```python
from build123d import *

# Parameters (mm, degrees)
SKETCH1_R                = 16.5
BOSS_EXTRUDE1_DEPTH      = 47.5
SKETCH2_R                = 14
BOSS_EXTRUDE2_DEPTH      = 4
SKETCH4_R                = 1.6
BOSS_EXTRUDE3_DEPTH      = 8
BOSS_EXTRUDE3_DEPTH_BACK = 1
SKETCH5_R                = 1.6
BOSS_EXTRUDE4_DEPTH      = 8
BOSS_EXTRUDE4_DEPTH_BACK = 1


with BuildPart() as part:
    # Sketch1 → Boss-Extrude1 (new body)
    with BuildSketch(Plane(origin=(0, 0, 0), x_dir=(1, 0, 0), z_dir=(0, 1, 0))):
        Circle(SKETCH1_R)
    extrude(amount=BOSS_EXTRUDE1_DEPTH)

    # Sketch2 → Boss-Extrude2 (add)
    with BuildSketch(Plane.XZ):
        Circle(SKETCH2_R)
    extrude(amount=BOSS_EXTRUDE2_DEPTH)

    # Sketch4 → Boss-Extrude3 (add, two sides)
    with BuildSketch(Plane(origin=(0, 0, -16.5), x_dir=(-1, 0, 0), z_dir=(0, 0, -1))) as boss_extrude3_sk:
        with Locations((0, 35.800460913)):
            Circle(SKETCH4_R)
        with Locations((0, 13.800460913)):
            Circle(SKETCH4_R)
    extrude(amount=BOSS_EXTRUDE3_DEPTH)
    extrude(boss_extrude3_sk.sketch, amount=-BOSS_EXTRUDE3_DEPTH_BACK)

    # Sketch5 → Boss-Extrude4 (add, two sides)
    with BuildSketch(Plane(origin=(16.5, 0, 0), x_dir=(0, 0, -1), z_dir=(1, 0, 0))) as boss_extrude4_sk:
        with Locations((0, 20)):
            Circle(SKETCH5_R)
    extrude(amount=BOSS_EXTRUDE4_DEPTH)
    extrude(boss_extrude4_sk.sketch, amount=-BOSS_EXTRUDE4_DEPTH_BACK)


solid = part.part
```
Source: CAD feature listing. Evaluate the final solid. Frame: model axes, mm. A direction names the side the tool comes from. Give positions to 0.01 mm unless a question says otherwise; leave off trailing zeros. Order: outer loops, then holes, each group sorted by start corner. A loop starts at its lowest first (then second) coordinate and runs counter-clockwise, first axis right, second up.
(1) Section query B-B (y = 1). Return the cut outline in (x, z), plus the area to 3 significant figures.
(2) Section query A-A (z = -5.5). Return the cut outline in (x, y), plus the area to 3 significant figures.
(3) Section query D-D (z = -18.5). Return the cut outline in (x, y), plus the area to 3 significant figures.
(4) Contact query for flat-ended pins moving along their axis: P1, Ø12, axis at x = 1.5, y = 17, coming from the +Z side; P2, Ø3, axis at x = 0, y = 28.5, coming from the -Z side; P3, Ø4, axis at y = 10, z = -12.5, coming from the -X side; P4, Ø12, axis at y = 31.5, z = 11, coming from the +X side. Output: stop coordinate, or through.
(5) Section query C-C (x = 6). Return the cut outline in (y, z), plus the area to 3 significant figures.
(6) Material intervals for line 1 along Y through (x, z) = (7, -14); line 2 along Y through (x, z) = (-1, -23); line 3 along X through (y, z) = (14, -3), sorted ascending.
(7) Access query for faces 1 (the face through (0, 47.5, 0)), 2 (the face through (-7.4, 0, 12.1)). Directions: +Z, -Z, +X, -X, +Y, -Y. A direction counts if a zero-diameter tool reaches every point of the face in a straight line with its end or side. Return the directions, or none.
Outcome:
1. outline: circle Ø33 at (0, 0)
1. area: 855 mm2
2. outline: (-15.56, 0) - (-12.87, 0) - (-12.87, -4) - (12.87, -4) - (12.87, 0) - (15.56, 0) - (15.56, 47.5) - (-15.56, 47.5) - close
2. area: 1,580 mm2
3. outline: circle Ø3.2 at (0, 13.8); circle Ø3.2 at (0, 35.8)
3. area: 16.1 mm2
4. P1: stops at z = 16.5
4. P2: stops at z = -16.5
4. P3: stops at x = -12.73
4. P4: stops at x = 15.72
5. outline: (-4, -12.65) - (0, -12.65) - (0, -15.37) - (47.5, -15.37) - (47.5, 15.37) - (0, 15.37) - (0, 12.65) - (-4, 12.65) - close
5. area: 1,560 mm2
6. line 1: y = 0 to 47.5
6. line 2: y = 12.55 to 15.05, 34.55 to 37.05
6. line 3: x = -16.22 to 16.22
7. face 1: +Z, -Z, +X, -X, +Y
7. face 2: -Y
